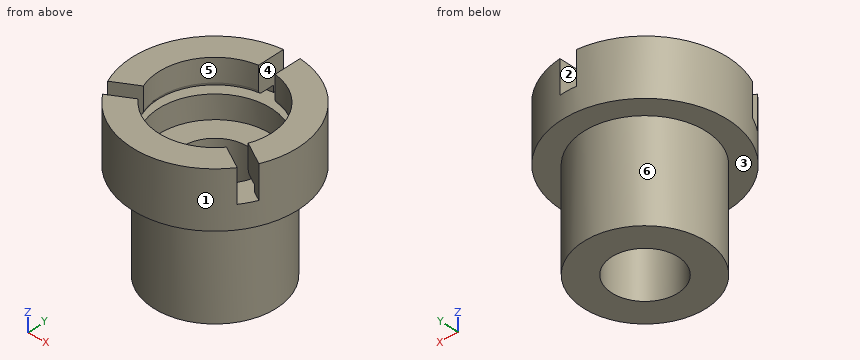
from build123d import *

# Parameters (mm, degrees)
SKETCH_1_R          = 1.85
SKETCH_1_R_2        = 1
EXTRUDE_3_DEPTH     = 3
SKETCH_4_R          = 2.5
SKETCH_4_R_2        = 1.7
EXTRUDE_4_DEPTH     = 1.7
CUT_EXTRUDE_3_DEPTH = 1
SKETCH_7_W          = 0.2
SKETCH_7_H          = 0.5
FILLET_1_R          = 0.1


with BuildPart() as part:
    # Эскиз1 → Бобышка-Вытянуть3 (new body)
    with BuildSketch(Plane.XY):
        Circle(SKETCH_1_R)
        Circle(SKETCH_1_R_2, mode=Mode.SUBTRACT)
    extrude(amount=EXTRUDE_3_DEPTH)

    # Эскиз4 → Бобышка-Вытянуть4 (add)
    with BuildSketch(Plane.XY.offset(3)):
        Circle(SKETCH_4_R)
        Circle(SKETCH_4_R_2, mode=Mode.SUBTRACT)
    extrude(amount=EXTRUDE_4_DEPTH)

    # Эскиз5 → Вырез-Вытянуть3 (cut)
    with BuildSketch(Plane.XY.offset(4.7)):
        with BuildLine():
            Line((0.25, 1.580348063), (0.25, 2.5))
            ThreePointArc((0.25, 2.5), (0, 2.512468905), (-0.25, 2.5))
            Line((-0.25, 2.5), (-0.25, 1.580348063))
            ThreePointArc((-0.25, 1.580348063), (0, 1.6), (0.25, 1.580348063))
        make_face()
        with BuildLine():
            Line((1.243621569, -1.006680382), (2.040063509, -1.466506351))
            ThreePointArc((2.040063509, -1.466506351), (2.175861898, -1.256234453), (2.290063509, -1.033493649))
            Line((2.290063509, -1.033493649), (1.493621569, -0.573667681))
            ThreePointArc((1.493621569, -0.573667681), (1.385640646, -0.8), (1.243621569, -1.006680382))
        make_face()
        with BuildLine():
            Line((-1.493621569, -0.573667681), (-2.290063509, -1.033493649))
            ThreePointArc((-2.290063509, -1.033493649), (-2.175861898, -1.256234453), (-2.040063509, -1.466506351))
            Line((-2.040063509, -1.466506351), (-1.243621569, -1.006680382))
            ThreePointArc((-1.243621569, -1.006680382), (-1.385640646, -0.8), (-1.493621569, -0.573667681))
        make_face()
    extrude(amount=-CUT_EXTRUDE_3_DEPTH, mode=Mode.SUBTRACT)

    # Эскиз7 → Вырез-Повернуть1 (revolve, cut)
    with BuildSketch(Plane(origin=(0, 0, 0), x_dir=(0, 0, -1), z_dir=(1, 0, 0)), mode=Mode.PRIVATE) as cut_revolve_1_sk:
        with Locations((-3.8, 1.931517172)):
            Rectangle(SKETCH_7_W, SKETCH_7_H)
    revolve(cut_revolve_1_sk.sketch.rotate(Axis((0, 0, 0), (0, 0, 1)), 270), axis=Axis((0, 0, 0), (0, 0, 1)), mode=Mode.SUBTRACT)

    # Скругление1
    fillet_1_edges = [part.edges().sort_by_distance(p)[0] for p in [
        (0, -1.7, 3.9),
        (1.472243186, 0.85, 3.9),
        (-1.472243186, 0.85, 3.9),
    ]]
    fillet(fillet_1_edges, radius=FILLET_1_R)


solid = part.part
Can you work these out from the model? Positions are in its coordinate system, mm. Face numbers are marked on the shaded views. A direction names the side the tool comes from. Round coordinates to 2 decimals unless told otherwise and drop trailing zeros. Order: outer loops, then holes, each group sorted by start corner. A loop starts at its lowest first (then second) coordinate and runs counter-clockwise, first axis right, second up. Notation, with made-up numbers: (-22.75, 52) - (-0.75, 52) arc R19 ccw to (-0.75, 69) - close; hole circle Ø1 at (42.25, 28.25). An arc over 180 degrees is marked (long way). Answer in a Markdown table with one row per item.
(1) Please list where these lines run through material, in increasing order: L1, parallel to Y at x = 0, z = 3.55; L2, parallel to Y at x = 0, z = 1.1. Write a range as from..to.
From the geometry:
| item | result |
|---|---|
| L1 | y = -2.5..-1.7, 1.7..2.5 |
| L2 | y = -1.85..-1, 1..1.85 |
(2) Suppose I cut it at A-A, the plane y = 0. Please give me the cut outline in (x, z), plus the area to 3 significant figures.
From the geometry:
| item | result |
|---|---|
| outline | (-2.5, 3) - (-1.85, 3) - (-1.85, 0) - (-1, 0) - (-1, 3) - (-1.7, 3) - (-1.7, 3.7) - (-2.18, 3.7) - (-2.18, 3.9) - (-1.8, 3.9) arc R0.1 ccw to (-1.7, 4) - (-1.7, 4.7) - (-2.5, 4.7) - close; (1, 0) - (1.85, 0) - (1.85, 3) - (2.5, 3) - (2.5, 4.7) - (1.7, 4.7) - (1.7, 4) arc R0.1 ccw to (1.8, 3.9) - (2.18, 3.9) - (2.18, 3.7) - (1.7, 3.7) - (1.7, 3) - (1, 3) - close |
| area | 7.62 mm2 |
(3) If we mould it in two halves opening along X, with no side actions, what happens to the marked faces 1, 2 and 3? For each: released by +X, released by -X, zero draft, split by the parting line, or undercut.
From the geometry:
| item | result |
|---|---|
| face 1 | split by the parting line |
| face 2 | undercut |
| face 3 | zero draft |
(4) Suppose I cut it at B-B, the plane x = 0. Please give me the cut outline in (y, z).
From the geometry:
| item | result |
|---|---|
| outline | (-2.5, 3) - (-1.85, 3) - (-1.85, 0) - (-1, 0) - (-1, 3) - (-1.7, 3) - (-1.7, 3.7) - (-2.18, 3.7) - (-2.18, 3.9) - (-1.8, 3.9) arc R0.1 ccw to (-1.7, 4) - (-1.7, 4.7) - (-2.5, 4.7) - close; (1, 0) - (1.85, 0) - (1.85, 3) - (2.5, 3) - (2.5, 3.7) - (1.7, 3.7) - (1.7, 3) - (1, 3) - close |
(5) Suppose I cut it at C-C, the plane z = 1.95. Please give me the cut outline in (x, y).
From the geometry:
| item | result |
|---|---|
| outline | circle Ø3.7 at (0, 0); hole circle Ø2 at (0, 0) |
(6) Which directions (+Z, -Z, +X, -X, +Y, -Y) give clear straight access to the entire face, cutting with the end or side of a thin tool? Please do the marked faces 4, 5 and 6.
From the geometry:
| item | result |
|---|---|
| face 4 | +Z, +Y |
| face 5 | +Z |
| face 6 | -Z |
(7) For P1, Ø2.5, axis at x = 0, y = 0, coming from the +Z side; P2, Ø1, axis at x = 0.5, z = 1, coming from the -Y side; P3, Ø1, axis at y = -0.5, z = 1, coming from the +X side, each with a flat end and sliding along its axis, tell me the tip position at first contact or that it passes through.
From the geometry:
| item | result |
|---|---|
| P1 | stops at z = 3 |
| P2 | stops at y = -1.85 |
| P3 | stops at x = 1.85 |
(8) Suppose I cut it at D-D, the plane y = -2.05. Please give me the cut outline in (x, z).
From the geometry:
| item | result |
|---|---|
| outline | (-1.43, 3) - (1.43, 3) - (1.43, 4.7) - (-1.43, 4.7) - close; hole (-0.75, 3.7) - (0.75, 3.7) - (0.75, 3.9) - (-0.75, 3.9) - close |
